Geometry check sheet. Reference: the model listing, model coordinates, mm. Coordinates: 2 decimals unless noted, no trailing zeros. Order: outer loops, then holes, each group sorted by start corner. A loop starts at its lowest first (then second) coordinate and runs counter-clockwise, first axis right, second up. Notation, with made-up numbers: (59.25, 49.25) - (118.25, 49.25) arc R18 ccw to (118.25, 53.25) - close; hole circle Ø6 at (-28, 69.25). An arc over 180 degrees is marked (long way). Use CSV: the item, a comma, the result in double quotes. Start each with the question number.
1) Thickness scan on probe 1 along X at (y, z) = (-8, -1.1); probe 2 along Y at (x, z) = (-31.96, -0.85); probe 3 along X at (y, z) = (-9, -0.9). Record the ranges inside material, lowest first. Write a range as [from, to].
2) Sectioned sample at D-D, the plane y = 45. Record the cut outline in (x, z), and give its area (3 significant figures).
3) Sectioned sample at B-B, the plane x = 10. Record the cut outline in (y, z).
4) Sectioned sample at C-C, the plane z = -0.6. Record the cut outline in (x, y), and give its area (3 significant figures).
5) Sectioned sample at A-A, the plane y = -10. Record the cut outline in (x, z), and give its area (3 significant figures).
from build123d import *

# Parameters (mm, degrees)
BASE_FLANGE1_DEPTH   = 2
M5_CLEARANCE_HOLE2_D = 5.5
BREAK_CORNER1_START  = -2
BREAK_CORNER1_DEPTH  = 2


# Read off the part's stored shape, not the designer's step: Break-Corner1
# Sheet-metal steps are written as plain solids
with BuildPart() as part:
    # Sketch2 → Base-Flange1 (new body)
    with BuildSketch(Plane.XY):
        Polygon((0, 60), (-103.923048454, 0), (-103.923048454, -20), (20, -20), (20, 0), (20, 60), align=None)
    extrude(amount=-BASE_FLANGE1_DEPTH)

    # M5 Clearance Hole2 (through all)
    with Locations(Plane.XY):
        with Locations((-88.923048454, -10), (-31.96, -10), (10, 10), (10, 45)):
            Hole(M5_CLEARANCE_HOLE2_D / 2)

    # Break-Corner1 outline → Break-Corner1 (cut)
    with BuildSketch(Plane.XY.offset(BREAK_CORNER1_START)):
        with BuildLine():
            ThreePointArc((17.5, 60), (19.267766953, 59.267766953), (20, 57.5))
            Line((20, 57.5), (20, 60))
            Line((20, 60), (17.5, 60))
        make_face()
        with BuildLine():
            Line((20, -20), (20, -17.5))
            ThreePointArc((20, -17.5), (19.267766953, -19.267766953), (17.5, -20))
            Line((17.5, -20), (20, -20))
        make_face()
        with BuildLine():
            ThreePointArc((-0.580127019, 59.665063509), (0.022825368, 59.914814566), (0.669872981, 60))
            Line((0.669872981, 60), (0, 60))
            Line((0, 60), (-0.580127019, 59.665063509))
        make_face()
        with BuildLine():
            Line((-103.923048454, -20), (-101.423048454, -20))
            ThreePointArc((-101.423048454, -20), (-103.190815407, -19.267766953), (-103.923048454, -17.5))
            Line((-103.923048454, -17.5), (-103.923048454, -20))
        make_face()
        with BuildLine():
            ThreePointArc((-103.923048454, -1.443375673), (-103.588111964, -0.193375673), (-102.673048454, 0.721687836))
            Line((-102.673048454, 0.721687836), (-103.923048454, 0))
            Line((-103.923048454, 0), (-103.923048454, -1.443375673))
        make_face()
    extrude(amount=BREAK_CORNER1_DEPTH, mode=Mode.SUBTRACT)


solid = part.part
Evaluation:
1,probe 1,"[-103.92, -90.81], [-87.04, -33.85], [-30.07, 20]"
1,probe 2,"[-20, -12.75], [-7.25, 41.55]"
1,probe 3,"[-103.92, -91.48], [-86.36, -34.52], [-29.4, 20]"
2,outline,"(-25.98, -2) - (7.25, -2) - (7.25, 0) - (-25.98, 0) - close; (12.75, -2) - (20, -2) - (20, 0) - (12.75, 0) - close"
2,area,"81.0 mm²"
3,outline,"(-20, -2) - (7.25, -2) - (7.25, 0) - (-20, 0) - close; (12.75, -2) - (42.25, -2) - (42.25, 0) - (12.75, 0) - close; (47.75, -2) - (60, -2) - (60, 0) - (47.75, 0) - close"
4,outline,"(-103.92, -17.5) arc R2.5 ccw to (-101.42, -20) - (17.5, -20) arc R2.5 ccw to (20, -17.5) - (20, 57.5) arc R2.5 ccw to (17.5, 60) - (0.67, 60) arc R2.5 ccw to (-0.58, 59.67) - (-102.67, 0.72) arc R2.5 ccw to (-103.92, -1.44) - close; hole circle Ø5.5 at (-88.92, -10); hole circle Ø5.5 at (-31.96, -10); hole circle Ø5.5 at (10, 10); hole circle Ø5.5 at (10, 45)"
4,area,"6,700 mm²"
5,outline,"(-103.92, -2) - (-91.67, -2) - (-91.67, 0) - (-103.92, 0) - close; (-86.17, -2) - (-34.71, -2) - (-34.71, 0) - (-86.17, 0) - close; (-29.21, -2) - (20, -2) - (20, 0) - (-29.21, 0) - close"
5,area,"226 mm²"
